Check sheet for the modelled part. Datum: model origin and axes. Units: mm. Give positions to 0.01 mm unless a question says otherwise; leave off trailing zeros. Loops run counter-clockwise (first coordinate to the right, second up) from the corner with the lowest first, then second, coordinate; pieces in that order, holes last. Notation, with made-up numbers: (79.25, 14) - (113.25, 14) arc R11 cw to (113.25, 21) - close; hole circle Ø8 at (-24, 2). An arc over 180 degrees is marked (long way). Use one line per item in the form item = value.
from build123d import *

# Parameters (mm, degrees)
SKETCH_1_W          = 56
SKETCH_1_H          = 25
EXTRUDE_1_DEPTH     = 2
SKETCH_2_R          = 4
SKETCH_2_R_2        = 1.5
CUT_EXTRUDE_1_DEPTH = 39.082744359
EXTRUDE_2_DEPTH     = 2
CUT_EXTRUDE_2_REACH = 74.741
SKETCH_4_R          = 4
SKETCH_4_R_2        = 1.5


with BuildPart() as part:
    # Sketch 1 → Extrude 1 (new body)
    with BuildSketch(Plane(origin=(0, 0, 0), x_dir=(1, 0, 0), z_dir=(0, 1, 0))):
        with Locations((7.654255319, 0.731382979)):
            Rectangle(SKETCH_1_W, SKETCH_1_H)
    extrude(amount=EXTRUDE_1_DEPTH)

    # Sketch 2 → Cut-Extrude 1 (cut, through all)
    with BuildSketch(Plane(origin=(0, 2, 0), x_dir=(1, 0, 0), z_dir=(0, 1, 0))):
        with Locations(Location((7.654255319, 0.731382979, 0), (0, 0, 270))):
            Circle(SKETCH_2_R)
        with Locations(Location((7.654255319, 7.731382979, 0), (0, 0, 270))):
            Circle(SKETCH_2_R_2)
        with Locations(Location((14.654255319, 0.731382979, 0), (0, 0, 270))):
            Circle(SKETCH_2_R_2)
        with Locations(Location((7.654255319, -6.268617021, 0), (0, 0, 270))):
            Circle(SKETCH_2_R_2)
        with Locations(Location((0.654255319, 0.731382979, 0), (0, 0, 270))):
            Circle(SKETCH_2_R_2)
        with Locations(Location((-10.945744681, 0.731382979, 0), (0, 0, 270))):
            Circle(SKETCH_2_R_2)
        with Locations(Location((26.254255319, 0.731382979, 0), (0, 0, 270))):
            Circle(SKETCH_2_R_2)
    extrude(amount=-CUT_EXTRUDE_1_DEPTH, mode=Mode.SUBTRACT)

    # Sketch 3 → Extrude 2 (add)
    with BuildSketch(Plane.ZY.offset(20.345744681)):
        with BuildLine():
            Line((-13.231382979, 2), (11.768617021, 2))
            Line((11.768617021, 2), (11.768617021, 32))
            ThreePointArc((11.768617021, 32), (-0.731382979, 44.5), (-13.231382979, 32))
            Line((-13.231382979, 32), (-13.231382979, 2))
        make_face()
    extrude_2 = extrude(amount=-EXTRUDE_2_DEPTH)

    # Sketch 4 → Cut-Extrude 2 (cut, up to next)
    with BuildSketch(Plane.ZY.offset(20.345744681), mode=Mode.PRIVATE) as cut_extrude_2_sk1:
        with Locations((-0.731382979, 32)):
            Circle(SKETCH_4_R)
    cut_extrude_2_tool1 = extrude(cut_extrude_2_sk1.sketch, amount=-CUT_EXTRUDE_2_REACH, mode=Mode.PRIVATE) & part.part
    # Sketch 4 → Cut-Extrude 2 (cut, up to next)
    with BuildSketch(Plane.ZY.offset(20.345744681), mode=Mode.PRIVATE) as cut_extrude_2_sk2:
        with Locations((-0.731382979, 39)):
            Circle(SKETCH_4_R_2)
    cut_extrude_2_tool2 = extrude(cut_extrude_2_sk2.sketch, amount=-CUT_EXTRUDE_2_REACH, mode=Mode.PRIVATE) & part.part
    # Sketch 4 → Cut-Extrude 2 (cut, up to next)
    with BuildSketch(Plane.ZY.offset(20.345744681), mode=Mode.PRIVATE) as cut_extrude_2_sk3:
        with Locations((6.268617021, 32)):
            Circle(SKETCH_4_R_2)
    cut_extrude_2_tool3 = extrude(cut_extrude_2_sk3.sketch, amount=-CUT_EXTRUDE_2_REACH, mode=Mode.PRIVATE) & part.part
    # Sketch 4 → Cut-Extrude 2 (cut, up to next)
    with BuildSketch(Plane.ZY.offset(20.345744681), mode=Mode.PRIVATE) as cut_extrude_2_sk4:
        with Locations((-0.731382979, 25)):
            Circle(SKETCH_4_R_2)
    cut_extrude_2_tool4 = extrude(cut_extrude_2_sk4.sketch, amount=-CUT_EXTRUDE_2_REACH, mode=Mode.PRIVATE) & part.part
    # Sketch 4 → Cut-Extrude 2 (cut, up to next)
    with BuildSketch(Plane.ZY.offset(20.345744681), mode=Mode.PRIVATE) as cut_extrude_2_sk5:
        with Locations((-7.731382979, 32)):
            Circle(SKETCH_4_R_2)
    cut_extrude_2_tool5 = extrude(cut_extrude_2_sk5.sketch, amount=-CUT_EXTRUDE_2_REACH, mode=Mode.PRIVATE) & part.part
    # Sketch 4 → Cut-Extrude 2 (cut, up to next)
    with BuildSketch(Plane.ZY.offset(20.345744681), mode=Mode.PRIVATE) as cut_extrude_2_sk6:
        with Locations((-0.731382979, 13.4)):
            Circle(SKETCH_4_R_2)
    cut_extrude_2_tool6 = extrude(cut_extrude_2_sk6.sketch, amount=-CUT_EXTRUDE_2_REACH, mode=Mode.PRIVATE) & part.part
    cut_extrude_2_1 = cut_extrude_2_tool1.solids().sort_by_distance((-20.345745, 32, -0.731383))[0]
    add(cut_extrude_2_1, mode=Mode.SUBTRACT)
    cut_extrude_2_2 = cut_extrude_2_tool2.solids().sort_by_distance((-20.345745, 39, -0.731383))[0]
    add(cut_extrude_2_2, mode=Mode.SUBTRACT)
    cut_extrude_2_3 = cut_extrude_2_tool3.solids().sort_by_distance((-20.345745, 32, 6.268617))[0]
    add(cut_extrude_2_3, mode=Mode.SUBTRACT)
    cut_extrude_2_4 = cut_extrude_2_tool4.solids().sort_by_distance((-20.345745, 25, -0.731383))[0]
    add(cut_extrude_2_4, mode=Mode.SUBTRACT)
    cut_extrude_2_5 = cut_extrude_2_tool5.solids().sort_by_distance((-20.345745, 32, -7.731383))[0]
    add(cut_extrude_2_5, mode=Mode.SUBTRACT)
    cut_extrude_2_6 = cut_extrude_2_tool6.solids().sort_by_distance((-20.345745, 13.4, -0.731383))[0]
    add(cut_extrude_2_6, mode=Mode.SUBTRACT)
    cut_extrude_2 = cut_extrude_2_1 + cut_extrude_2_2 + cut_extrude_2_3 + cut_extrude_2_4 + cut_extrude_2_5 + cut_extrude_2_6  # Cut-Extrude 2 as one shape, for the pattern or mirror that repeats it

    # Mirror 1: Extrude 2, Cut-Extrude 2 across plane
    add(extrude_2.mirror(Plane.ZY.offset(-7.654255319)))
    add(cut_extrude_2.mirror(Plane.ZY.offset(-7.654255319)), mode=Mode.SUBTRACT)


solid = part.part
Item 1: Gauge pin test, flat end, axial feed: P1, Ø5, axis at x = 0.65, z = -0.73, coming from the +Y side. Record the tip position at first contact, or that the pin passes through.
Answer block:
P1 = 2
Item 2: Section check D-D on x = -3.5. Record the boundary of the cut face in (y, z), then the cut area to 3 significant figures.
Answer block:
outline = (0, -13.23) - (2, -13.23) - (2, 11.77) - (0, 11.77) - close
area = 50.0 mm2
Item 3: Section check A-A on y = 9. Record the boundary of the cut face in (x, z), then the cut area to 3 significant figures.
Answer block:
outline = (-20.35, -13.23) - (-18.35, -13.23) - (-18.35, 11.77) - (-20.35, 11.77) - close; (33.65, -13.23) - (35.65, -13.23) - (35.65, 11.77) - (33.65, 11.77) - close
area = 100 mm2
Item 4: Thickness scan on L1, parallel to X at y = 4, z = 8.5; L2, parallel to Y at x = -6, z = 1. Record the ranges inside material, lowest first.
Answer block:
L1 = -20.35 to -18.35, 33.65 to 35.65
L2 = 0 to 2
Item 5: Section check B-B on y = 25. Record the boundary of the cut face in (x, z).
Answer block:
outline = (-20.35, -13.23) - (-18.35, -13.23) - (-18.35, -2.23) - (-20.35, -2.23) - close; (-20.35, 0.77) - (-18.35, 0.77) - (-18.35, 11.77) - (-20.35, 11.77) - close; (33.65, -13.23) - (35.65, -13.23) - (35.65, -2.23) - (33.65, -2.23) - close; (33.65, 0.77) - (35.65, 0.77) - (35.65, 11.77) - (33.65, 11.77) - close
Item 6: Mould release check, pull along Z, two halves, no side actions. Record for faces 1 (the face through (-19.36, 26.487, -0.927)), 2 (the face through (8, 1, -13.231)), 3 (the face through (-19.36, 44.497, -0.457)): released by +Z, released by -Z, zero draft, split by the parting line, or undercut.
Answer block:
face_1 = undercut
face_2 = released by -Z
face_3 = split by the parting line
Item 7: Section check C-C on x = 7. Record the boundary of the cut face in (y, z).
Answer block:
outline = (0, -13.23) - (2, -13.23) - (2, -9.08) - (0, -9.08) - close; (0, -6.38) - (2, -6.38) - (2, -4.68) - (0, -4.68) - close; (0, 3.21) - (2, 3.21) - (2, 4.92) - (0, 4.92) - close; (0, 7.62) - (2, 7.62) - (2, 11.77) - (0, 11.77) - close
